Answer from the drawing. Dimensions are ordinates in mm from the lowest x, y and z of the part. A direction names the side the tool comes from. Give positions to 0.01 mm unless a question says otherwise; leave off trailing zeros. Loops run counter-clockwise (first coordinate to the right, second up) from the corner with the lowest first, then second, coordinate; pieces in that order, holes last. Notation, with made-up numbers: (-36, 64.25) - (13, 64.25) arc R16 ccw to (13, 93.25) - close; hole circle Ø8 at (83, 88.25). An arc over 180 degrees is marked (long way). Answer as CSV lines item,"result". Start each with the question number.
1) A cutting plane is placed at C-C (z = 6). Determine the outline of the cut face in (x, y).
2) Find the intervals of material crossed by line 1 along Z through (x, y) = (4.7, 3.8); line 2 along Y through (x, z) = (3.5, 6.75); line 3 along X through (y, z) = (4.5, 6.25), in increasing order.
3) Flat-ended cylindrical pins translate along their axes: pin 1 (3.5 mm diameter, centred on x = 4, y = 1, fed in from -Z); pin 2 (5 mm diameter, centred on y = 7.5, z = 4, fed in from +X); pin 3 (3 mm diameter, centred on y = 6, z = 5, fed in from -X). Find the tip coordinate at first contact, or state that the pin passes through.
4) For the marked faces 5, 6, 7, 8 and 9, determine the directions among +Z, -Z, +X, -X, +Y, -Y from which every point of the face is accessible in a straight line to the end or side of a thin tool.
5) For a pull along Z with two mould halves and no side action, classify the marked faces 1, 2, 3 and 4 as pulls with the +Z half, pulls with the -Z half, needs draft (parallel to the pull), parting line crosses it, or undercut.
6) A cutting plane is placed at D-D (x = 2.25). Determine the outline of the cut face in (y, z).
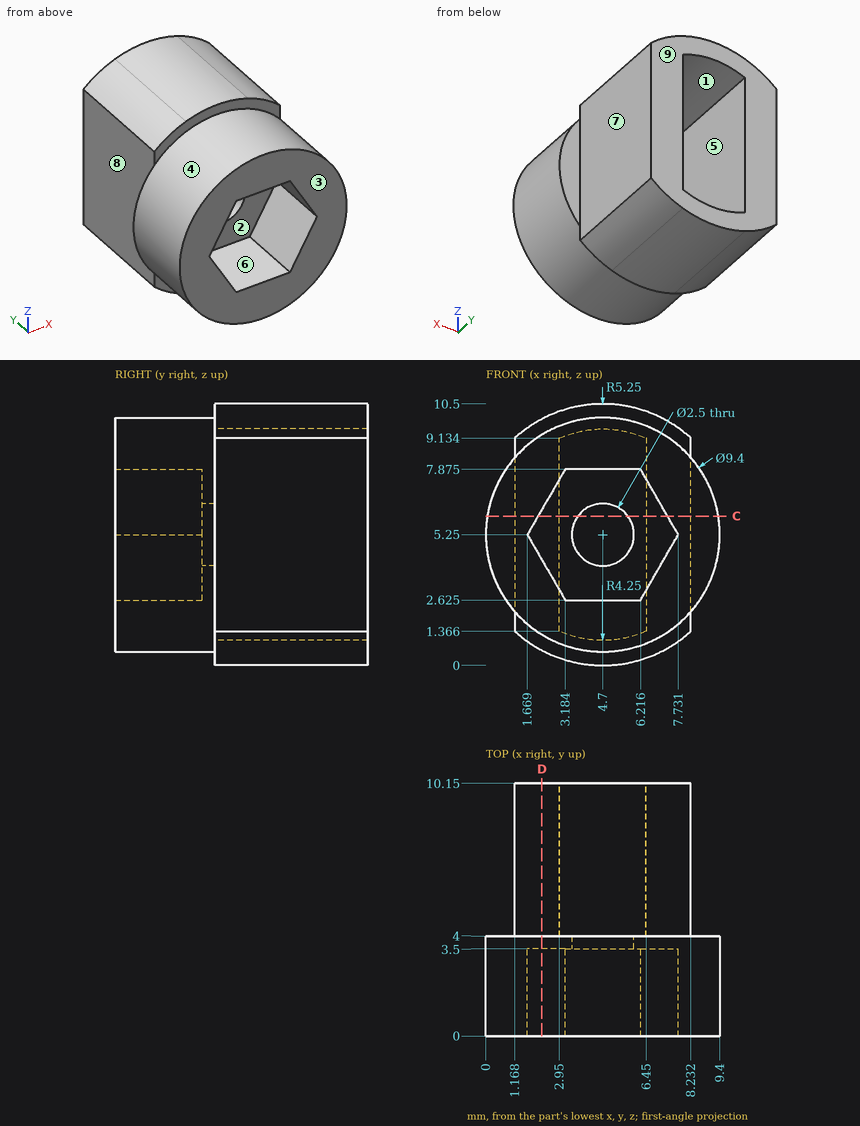
Ans:
1,outline,"(0.06, 0) - (2.1, 0) - (2.1, 3.5) - (3.7, 3.5) - (3.7, 4) - (2.95, 4) - (2.95, 10.15) - (1.17, 10.15) - (1.17, 4) - (0.06, 4) - close; (5.7, 3.5) - (7.3, 3.5) - (7.3, 0) - (9.34, 0) - (9.34, 4) - (8.23, 4) - (8.23, 10.15) - (6.45, 10.15) - (6.45, 4) - (5.7, 4) - close"
2,line 1,"0.55 to 4, 6.5 to 9.95"
2,line 2,"3.5 to 4"
2,line 3,"1.17 to 2.95, 6.45 to 8.23"
3,pin 1,"z = 0.55"
3,pin 2,"x = 8.23"
3,pin 3,"x = 1.17"
4,face 5,"+Y"
4,face 6,"-Y"
4,face 7,"+Z, -Z, +X, +Y"
4,face 8,"+Z, -Z, -X, +Y"
4,face 9,"+Z, -Z, +X, -X, +Y"
5,face 1,"undercut"
5,face 2,"undercut"
5,face 3,"needs draft"
5,face 4,"parting line crosses it"
6,outline,"(0, 1.24) - (4, 1.24) - (4, 0.61) - (10.15, 0.61) - (10.15, 9.89) - (4, 9.89) - (4, 9.26) - (0, 9.26) - (0, 6.26) - (3.5, 6.26) - (3.5, 4.24) - (0, 4.24) - close"
